For this review, use the dimensioned drawing (mm, ordinates from the lowest corner) and the shaded views. A direction names the side the tool comes from. Give positions to 0.01 mm unless a question says otherwise; leave off trailing zeros. Order: outer loops, then holes, each group sorted by start corner. A loop starts at its lowest first (then second) coordinate and runs counter-clockwise, first axis right, second up. Notation, with made-up numbers: M -17,13 L -10,13 A27 ccw -10,51 Z; hole C -12.5,-21.5 d3. An arc over 180 degrees is marked long. Answer as CSV lines item,"result". Start each with the question number.
1. We need section D-D, the plane z = 29.5. Give the boundary of the cut face in (x, y), and give its area (3 significant figures).
2. We need section B-B, the plane z = 18.5. Give the boundary of the cut face in (x, y), and give its area (3 significant figures).
3. Machinability: for the marked faces 4 and 5, which of the approach directions +Z, -Z, +X, -X, +Y, -Y give a long, thin tool a straight path to every point of the face, cutting with its end or side? Answer none if there is none.
4. Mouldability with a two-part tool opening along X and no side actions: class the marked faces 1, 2 and 3 as pulls with the +X half, pulls with the -X half, needs draft (parallel to the pull), parting line crosses it, or undercut.
5. For line 1 along X through (y, z) = (7, 18.5); line 2 along X through (y, z) = (11.75, 18.5); line 3 along Z through (x, y) = (20, 14.5), list the stretches that pass through material, from the lowest coordinate up.
6. We need section C-C, the plane y = 6.5. Give the boundary of the cut face in (x, z).
7. We need section A-A, the plane x = 18.5. Give the boundary of the cut face in (y, z), and give its area (3 significant figures).
8. Clearance check with flat-ended pins moving along their axes: P1, Ø6, axis at x = 18, y = 3.5, coming from the -Z side; P2, Ø3, axis at x = 29.5, y = 9.5, coming from the -Z side; P3, Ø4, axis at x = 4.5, z = 18, coming from the +Y side; P4, Ø8, axis at y = 9.5, z = 8.5, coming from the +X side. State where each tip first meets the part, or that it passes through.
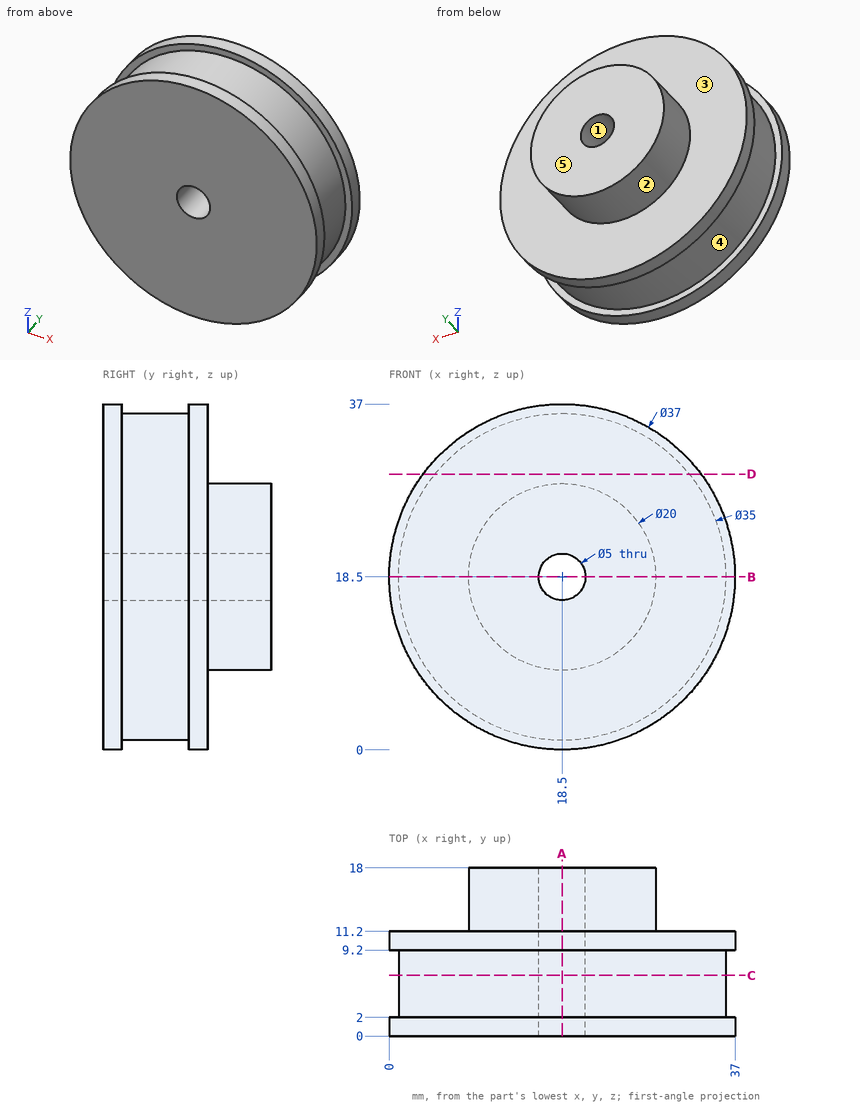
Result set:
1,outline,"M 3.63,0 L 33.37,0 L 33.37,2 L 32.11,2 L 32.11,9.2 L 33.37,9.2 L 33.37,11.2 L 3.63,11.2 L 3.63,9.2 L 4.89,9.2 L 4.89,2 L 3.63,2 Z"
1,area,"315 mm2"
2,outline,"M 0,0 L 16,0 L 16,18 L 8.5,18 L 8.5,11.2 L 0,11.2 L 0,9.2 L 1,9.2 L 1,2 L 0,2 Z; M 21,0 L 37,0 L 37,2 L 36,2 L 36,9.2 L 37,9.2 L 37,11.2 L 28.5,11.2 L 28.5,18 L 21,18 Z"
2,area,"446 mm2"
3,face 4,"none"
3,face 5,"+Z, -Z, +X, -X, +Y"
4,face 1,"undercut"
4,face 2,"parting line crosses it"
4,face 3,"needs draft"
5,line 1,"1 to 16, 21 to 36"
5,line 2,"8.5 to 16, 21 to 28.5"
5,line 3,"8.61 to 16.5, 20.5 to 28.39"
6,outline,"C 18.5,18.5 d35; hole C 18.5,18.5 d5"
7,outline,"M 0,0 L 2,0 L 2,1 L 9.2,1 L 9.2,0 L 11.2,0 L 11.2,8.5 L 18,8.5 L 18,16 L 0,16 Z; M 0,21 L 18,21 L 18,28.5 L 11.2,28.5 L 11.2,37 L 9.2,37 L 9.2,36 L 2,36 L 2,37 L 0,37 Z"
7,area,"446 mm2"
8,P1,"z = 0"
8,P2,"z = 2.63"
8,P3,"y = 11.2"
8,P4,"x = 36"
